```python
from build123d import *

# Parameters (mm, degrees)
F1_DEPTH = 24
F3_DEPTH = 7.001
F4_R     = 1.75
F5_DEPTH = 45.75


with BuildPart() as f1:
    # F0 (on Front) → F1 (new body, symmetric)
    with BuildSketch(Plane.XZ):
        with BuildLine():
            ThreePointArc((-16.406394, 4), (-18.010296, 1.816402), (-16, 0))
            Line((-16, 0), (16, 0))
            ThreePointArc((16, 0), (18.010296, 1.816402), (16.406394, 4))
            Line((16.406394, 4), (3.552904, 6.63903))
            ThreePointArc((3.552904, 6.63903), (0, 7), (-3.552904, 6.63903))
            Line((-3.552904, 6.63903), (-16.406394, 4))
        make_face()
    extrude(amount=F1_DEPTH, both=True)

    # F2 (on face) → F3 (cut, through all)
    with BuildSketch(Plane(origin=(0, 0, 0), x_dir=(1, 0, 0), z_dir=(0, 0, -1))):
        Polygon((-11, 19.5), (-11, -19.5), (-4, -19.5), (4, -19.5), (11, -19.5), (11, 19.5), (4, 19.5), (-4, 19.5), align=None)
    extrude(amount=-F3_DEPTH, mode=Mode.SUBTRACT)

    # F4 (on face) → F5 (cut, through all)
    with BuildSketch(Plane.XZ.offset(24)):
        with Locations((0, 3.5)):
            Circle(F4_R)
    extrude(amount=-F5_DEPTH, mode=Mode.SUBTRACT)


solid = f1.part
```
Could you check a few things on this model? Use its own coordinates, in mm. A direction names the side the tool comes from. Coordinates: 2 decimals unless noted, no trailing zeros. Write each loop counter-clockwise with the first axis right and the second up, starting at its lowest first coordinate (ties: lowest second). Pieces come first, ordered by that corner, then holes. Notation, with made-up numbers: M -27.5,22.25 L 23.5,22.25 A5 ccw 23.5,26.25 Z; hole C 79,-6 d7. An arc over 180 degrees is marked long. Answer as CSV lines item,"result". Start each with the question number.
1) For P1, Ø2, axis at x = 0, z = 3.5, coming from the -Y side, with a flat end and sliding along its axis, tell me the tip position at first contact or that it passes through.
2) For faces 4 (the cylindrical face through (-0.38, -21.78, 1.79)), 5 (the flat face through (-11, 0, 3)), 6 (the flat face through (14, 0, 0)), which set-ups out of +Z, -Z, +X, -X, +Y, -Y let a thin tool reach every point of the face, with its end or its side?
3) I want a section at B-B, the plane y = -8.5. Please give me the cut outline in (x, z), and give its area (3 significant figures).
4) I want a section at D-D, the plane z = 1. Please give me the cut outline in (x, y), and give its area (3 significant figures).
5) We'd pull the mould along Z, two halves only. Please class faces 1 (the flat face through (0, -24, 1)), 2 (the flat face through (0, 21.75, 4)), 3 (the cylindrical face through (0, -22, 7)): +Z half, -Z half, draft (parallel to the pull), parting line (faces both ways), or undercut.
6) I want a section at A-A, the plane x = 0. Please give me the cut outline in (y, z).
7) Please list where these lines run through material, in increasing order: line 1 (Y direction, x = -1.5, z = 2); line 2 (X direction, y = 7.5, z = 2); line 3 (Y direction, x = -1, z = 3.25). Write a range as from..to.
8) I want a section at C-C, the plane z = 6. Please give me the cut outline in (x, y).
Data:
1,P1,"stops at y = 21.75"
2,face 4,"-Y"
2,face 5,"+Z, -Z"
2,face 6,"-Z, +X, -X, +Y, -Y"
3,outline,"M -16.41,4 A2.02 ccw -16,0 L -11,0 L -11,5.11 Z; M 11,0 L 16,0 A2.02 ccw 16.41,4 L 11,5.11 Z"
3,area,"58.8 mm^2"
4,outline,"M -17.74,-24 L 17.74,-24 L 17.74,24 L -17.74,24 Z; hole M -11,-19.5 L 11,-19.5 L 11,19.5 L -11,19.5 Z"
4,area,"845 mm^2"
5,face 1,"draft"
5,face 2,"undercut"
5,face 3,"+Z half"
6,outline,"M -24,0 L -19.5,0 L -19.5,1.75 L -24,1.75 Z; M -24,5.25 L -19.5,5.25 L -19.5,7 L -24,7 Z; M 19.5,0 L 24,0 L 24,7 L 19.5,7 L 19.5,5.25 L 21.75,5.25 L 21.75,1.75 L 19.5,1.75 Z"
7,line 1,"y = -24..-19.5, 19.5..24"
7,line 2,"x = -18.02..-11, 11..18.02"
7,line 3,"y = 21.75..24"
8,outline,"M -6.67,-24 L 6.67,-24 L 6.67,-19.5 L -6.67,-19.5 Z; M -6.67,19.5 L 6.67,19.5 L 6.67,24 L -6.67,24 Z"
